Autodesk Inventor part; units mm, degrees
ref_plane "YZ Plane" through (0, 0, 0) normal (1, 0, 0) x (0, 1, 0)
ref_plane "XZ Plane" through (0, 0, 0) normal (0, 1, 0) x (-1, 0, 0)
ref_plane "XY Plane" through (0, 0, 0) normal (0, 0, 1) x (1, 0, 0)
sketch "Эскиз1" plane through (0, 0, 0) normal (0, 1, 0) x (-1, 0, 0)
  circle A0 centre (0, 0) radius 26
  dimension "d0" = 52
extrude "Выдавливание1" add sketch "Эскиз1" along normal blind 15
sketch "Эскиз2" plane through (0, 15, 0) normal (0, 1, 0) x (1, 0, 0)
  circle A0 centre (0, 0) radius 17.5
  circle A1 centre (0, 0) radius 12.5
  dimension "d3" = 25
  dimension "d4" = 35
extrude "Выдавливание2" add sketch "Эскиз2" along normal blind 12
sketch "Эскиз3" plane through (0, 0, 0) normal (0, -1, 0) x (1, 0, 0)
  circle A0 centre (0, 0) radius 12.5
  dimension "d7" = 25
extrude "Выдавливание3" cut sketch "Эскиз3" against normal blind 15
properties part number "подшипник"
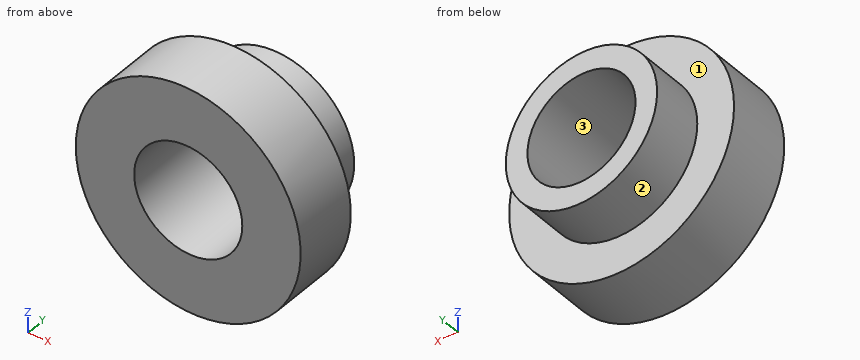
Can you work these out from the model? Positions are in its coordinate system, mm. Face numbers are marked on the shaded views. Give positions to 0.01 mm unless a question says otherwise; leave off trailing zeros. Loops run counter-clockwise (first coordinate to the right, second up) from the corner with the lowest first, then second, coordinate; pieces in that order, holes last. Notation, with made-up numbers: M -22,75.5 L 16,75.5 A22 ccw 16,86.5 Z; hole C 49,10.25 d1. An arc over 180 degrees is marked long. One line per item, written item: value.
(1) Suppose I cut it at A-A on z = 0. List the corners of the cut face in (x, y) for me.
Returned:
outline: M -26,0 L -12.5,0 L -12.5,27 L -17.5,27 L -17.5,15 L -26,15 Z; M 12.5,0 L 26,0 L 26,15 L 17.5,15 L 17.5,27 L 12.5,27 Z
(2) Will these pins go through, and if not, where does the flat tip stop? pin 1 (5 mm diameter, centred on x = 15, y = 14, fed in from -Z); pin 2 (22.5 mm diameter, centred on x = 0, z = 0, fed in from -Y); pin 3 (2 mm diameter, centred on x = 17, z = 9, fed in from -Y); pin 4 (8 mm diameter, centred on y = 8.5, z = -12, fed in from +X).
Returned:
pin 1: z = -22.8
pin 2: through
pin 3: y = 0
pin 4: x = 24.74
(3) We'd pull the mould along Z, two halves only. Please class the marked faces 1, 2 and 3: released by +Z, released by -Z, zero draft, split by the parting line, or undercut.
Returned:
face 1: zero draft
face 2: split by the parting line
face 3: undercut
(4) Suppose I cut it at D-D on x = -22. List the corners of the cut face in (y, z) for me, plus the area to 3 significant figures.
Returned:
outline: M 0,-13.86 L 15,-13.86 L 15,13.86 L 0,13.86 Z
area: 416 mm^2
(5) Suppose I cut it at C-C on y = 2.25. List the corners of the cut face in (x, z) for me, plus the area to 3 significant figures.
Returned:
outline: C 0,0 d52; hole C 0,0 d25
area: 1,630 mm^2
(6) I need wall thicknesses on line 1 (Z direction, x = 0, y = 13); line 2 (Z direction, x = 0, y = 20). Which ranges of each line are inside material? Lowest first, please.
Returned:
line 1: -26 to -12.5, 12.5 to 26
line 2: -17.5 to -12.5, 12.5 to 17.5
(7) Suppose I cut it at B-B on x = 0. List the corners of the cut face in (y, z) for me.
Returned:
outline: M 0,-26 L 15,-26 L 15,-17.5 L 27,-17.5 L 27,-12.5 L 0,-12.5 Z; M 0,12.5 L 27,12.5 L 27,17.5 L 15,17.5 L 15,26 L 0,26 Z
